Geometry: final body of the model. Coordinates: model frame, mm. Face numbers are marked on the shaded views. Round coordinates to 2 decimals unless told otherwise and drop trailing zeros. Order: outer loops, then holes, each group sorted by start corner. A loop starts at its lowest first (then second) coordinate and runs counter-clockwise, first axis right, second up. Notation, with made-up numbers: M -12,-32 L -4,-32 A23 cw -4,-5 Z; hole C 49.25,87.25 d10. An arc over 180 degrees is marked long. Return JSON: item names as keys, results as strings. Group by question number.
Q1. Mould query, pull axis Z, two halves, no side actions, for the marked faces 1, 2 and 3. Classes: released by +Z, released by -Z, zero draft, split by the parting line, or undercut.
Q2. Ray query, probe 1 along Z at (x, y) = (0, 3.75) (3 decimals); probe 2 along Z at (x, y) = (0, 10); probe 3 along Y at (x, z) = (-16, -10.5). Return the intervals inside material, ascending.
Q3. Contact query for flat-ended pins moving along their axis: pin 1 (3 mm diameter, centred on x = 0.5, y = 3, fed in from -Z) (3 decimals); pin 2 (8 mm diameter, centred on x = 7.5, y = 3, fed in from +Z); pin 3 (2 mm diameter, centred on x = -11.5, y = 8.5, fed in from -Z); pin 4 (7 mm diameter, centred on x = 0, z = 0, fed in from +Y). Output: stop coordinate, or through.
Q4. Cut plane C-C on y = 10.75. Output: boundary loops of the cut face in (x, z).
Q5. Cut plane D-D on x = -8. Output: boundary loops of the cut face in (y, z).
Q6. Cut plane B-B on x = 0. Output: boundary loops of the cut face in (y, z) (1 decimal), and give its area (4 significant figures).
Q7. Cut plane A-A on z = 0. Output: boundary loops of the cut face in (x, y) (1 decimal).
```python
from build123d import *

# Parameters (mm, degrees)
F0_R     = 27.5209
F1_DEPTH = 14.2875
F2_R     = 27.5209
F2_R_2   = 9.525
F3_DEPTH = 7.9375
F4_R     = 3.9624
F5_DEPTH = 14.2885


with BuildPart() as f1:
    # F0 (on Front) → F1 (new body)
    with BuildSketch(Plane.XZ):
        Circle(F0_R)
    extrude(amount=-F1_DEPTH)

    # F2 (on face) → F3 (cut)
    with BuildSketch(Plane.XZ):
        Circle(F2_R)
        Circle(F2_R_2, mode=Mode.SUBTRACT)
    extrude(amount=-F3_DEPTH, mode=Mode.SUBTRACT)

    # F4 (on face) → F5 (cut, through all)
    with BuildSketch(Plane.XZ):
        Circle(F4_R)
    extrude(amount=-F5_DEPTH, mode=Mode.SUBTRACT)


solid = f1.part
```
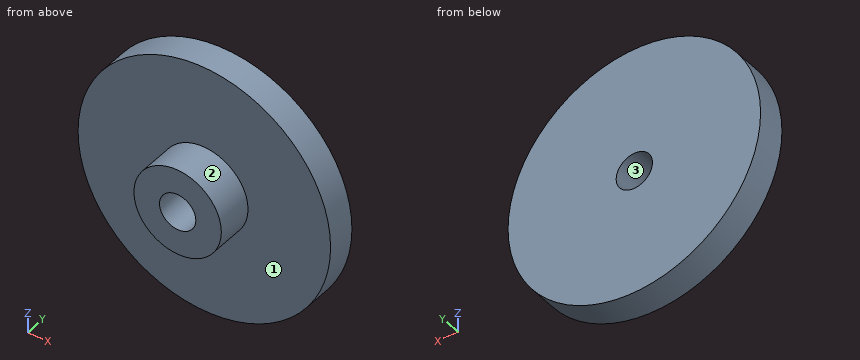
Result sheet:
{
 "1": {"face 1": "zero draft", "face 2": "split by the parting line", "face 3": "undercut"},
 "2": {"probe 1": "z = -9.525 to -3.962, 3.962 to 9.525", "probe 2": "z = -27.52 to -3.96, 3.96 to 27.52", "probe 3": "y = 7.94 to 14.29"},
 "3": {"pin 1": "stops at z = -9.525", "pin 2": "stops at z = 8.86", "pin 3": "stops at z = -25.44", "pin 4": "passes through"},
 "4": {"outline": "C 0,0 d55.04; hole C 0,0 d7.92"},
 "5": {"outline": "M 0,-5.17 L 7.94,-5.17 L 7.94,-26.33 L 14.29,-26.33 L 14.29,26.33 L 7.94,26.33 L 7.94,5.17 L 0,5.17 Z"},
 "6": {"outline": "M 0,-9.5 L 7.9,-9.5 L 7.9,-27.5 L 14.3,-27.5 L 14.3,-4 L 0,-4 Z; M 0,4 L 14.3,4 L 14.3,27.5 L 7.9,27.5 L 7.9,9.5 L 0,9.5 Z", "area": "387.5 mm²"},
 "7": {"outline": "M -27.5,7.9 L -9.5,7.9 L -9.5,0 L -4,0 L -4,14.3 L -27.5,14.3 Z; M 4,0 L 9.5,0 L 9.5,7.9 L 27.5,7.9 L 27.5,14.3 L 4,14.3 Z"}
}
